Verification items for the finished model (mm, model axes). Give positions to 0.01 mm unless a question says otherwise; leave off trailing zeros. Loops run counter-clockwise (first coordinate to the right, second up) from the corner with the lowest first, then second, coordinate; pieces in that order, holes last. Notation, with made-up numbers: (25.25, 14.5) -> (61.25, 14.5) arc R22 ccw to (61.25, 27.5) -> close; hole circle Ø6 at (57.25, -1). An arc over 180 degrees is marked (long way). Answer in a Markdown table with one row per item. Add a question column.
Q1. Material ranges on probe 1 along X at (y, z) = (0.25, 1.25); probe 2 along X at (y, z) = (-0.5, 0.15); probe 3 along Y at (x, z) = (150, 1.5), recorded low to high.
Q2. Section check A-A on z = 1.6. Enter the section's corners in (x, y), and give its area (3 significant figures).
Q3. Release check for a two-part mould opening along Y. For faces 1 (the face through (2, 0, 3)), 2 (the face through (-160, 0, 1)), 3 (the face through (-152.385, 0.751, 1.479)) record: pulls with the +Y half, pulls with the -Y half, needs draft (parallel to the pull), parting line crosses it, or undercut.
```python
from build123d import *

# Parameters (mm, degrees)
EXTRUDE_1_DEPTH     = 3
SKETCH_2_R          = 2.5
CUT_EXTRUDE_1_DEPTH = 3


with BuildPart() as part:
    # 草图1 → 凸台-拉伸1 (new body)
    with BuildSketch(Plane.XY):
        with BuildLine():
            Line((-150, 10), (150, 10))
            ThreePointArc((150, 10), (160, 0), (150, -10))
            Line((150, -10), (-150, -10))
            ThreePointArc((-150, -10), (-160, 0), (-150, 10))
        make_face()
    extrude(amount=EXTRUDE_1_DEPTH)

    # 草图2 → 切除-拉伸1 (cut)
    with BuildSketch(Plane(origin=(0, 0, 0), x_dir=(-1, 0, 0), z_dir=(0, 0, -1))):
        with Locations((150, 0)):
            Circle(SKETCH_2_R)
        with Locations((-150, 0)):
            Circle(SKETCH_2_R)
    extrude(amount=-CUT_EXTRUDE_1_DEPTH, mode=Mode.SUBTRACT)


solid = part.part
```
Taken from the geometry:
| question | item | result |
|---|---|---|
| 1 | probe 1 | x = -160 to -152.49, -147.51 to 147.51, 152.49 to 160 |
| 1 | probe 2 | x = -159.99 to -152.45, -147.55 to 147.55, 152.45 to 159.99 |
| 1 | probe 3 | y = -10 to -2.5, 2.5 to 10 |
| 2 | outline | (-150, -10) -> (150, -10) arc R10 ccw to (150, 10) -> (-150, 10) arc R10 ccw to start; hole circle Ø5 at (-150, 0); hole circle Ø5 at (150, 0) |
| 2 | area | 6,270 mm² |
| 3 | face 1 | needs draft |
| 3 | face 2 | parting line crosses it |
| 3 | face 3 | undercut |
